```python
from build123d import *

# Parameters (mm, degrees)
SKETCH_1_W              = 50
SKETCH_1_H              = 100
SKETCH_1_R              = 6.25
EXTRUDE_1_DEPTH         = 16
HOLE_WIZARD_M16_1_D     = 14
HOLE_WIZARD_M16_1_DEPTH = 38
HOLE_WIZARD_M16_1_TIP   = 4.206024333
SKETCH_5_R              = 9.25
CUT_EXTRUDE_1_DEPTH     = 12


with BuildPart() as part:
    # 草图1 → 凸台-拉伸1 (new body)
    with BuildSketch(Plane(origin=(0, 0, 0), x_dir=(1, 0, 0), z_dir=(0, 1, 0))):
        with Locations((25, 50)):
            Rectangle(SKETCH_1_W, SKETCH_1_H)
        with Locations(Location((25, 75, 0), (0, 0, 270))):
            Circle(SKETCH_1_R, mode=Mode.SUBTRACT)
        with Locations(Location((25, 25, 0), (0, 0, 270))):
            Circle(SKETCH_1_R, mode=Mode.SUBTRACT)
    extrude(amount=EXTRUDE_1_DEPTH)

    # M16 螺纹孔1
    with Locations(Plane(origin=(25, 16, -50), x_dir=(0, 0, 1), z_dir=(0, 1, 0))):
        with Locations((0, 0)):
            Hole(HOLE_WIZARD_M16_1_D / 2, depth=HOLE_WIZARD_M16_1_DEPTH)
            with Locations((0, 0, -(HOLE_WIZARD_M16_1_DEPTH + HOLE_WIZARD_M16_1_TIP / 2))):  # 118° drill point
                Cone(0, HOLE_WIZARD_M16_1_D / 2, HOLE_WIZARD_M16_1_TIP, mode=Mode.SUBTRACT)

    # 草图5 → 切除-拉伸1 (cut)
    with BuildSketch(Plane.XZ):
        with Locations(Location((25, -25, 0), (0, 0, 270))):
            Circle(SKETCH_5_R)
        with Locations(Location((25, -75, 0), (0, 0, 270))):
            Circle(SKETCH_5_R)
    extrude(amount=-CUT_EXTRUDE_1_DEPTH, mode=Mode.SUBTRACT)


solid = part.part
```
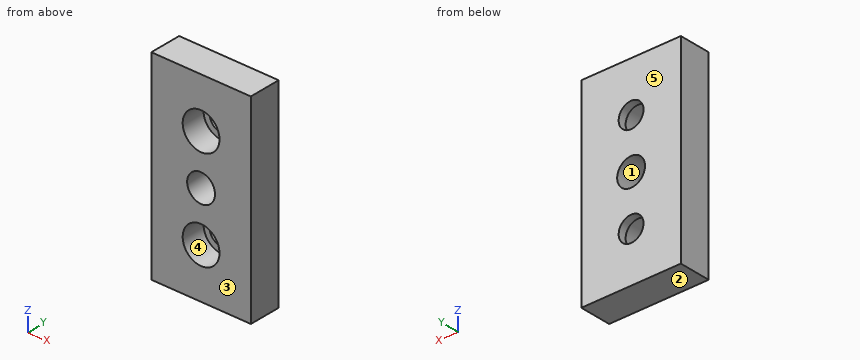
Model file for the job. Use its own axes, mm. Face numbers are marked on the shaded views. A direction names the side the tool comes from. Coordinates: 2 decimals unless noted, no trailing zeros. Order: outer loops, then holes, each group sorted by start corner. A loop starts at its lowest first (then second) coordinate and runs counter-clockwise, first axis right, second up. Notation, with made-up numbers: (-4.5, -33.75) -> (5.5, -33.75) arc R16 cw to (5.5, -11.75) -> close; hole circle Ø1 at (36.25, 16). An arc over 180 degrees is marked (long way). Answer as a JSON object with one key per item and string values. Group by question number.
1) Cut at C-C, the plane y = 10.5. Write the cut outline in (x, z), then the cut area to 3 significant figures.
2) Cut at B-B, the plane x = 25. Write the cut outline in (y, z), then the cut area to 3 significant figures.
3) Which spindle directions (+Z, -Z, +X, -X, +Y, -Y) get a long thin tool onto all of the face, cutting with end or side? Do the marked faces 4 and 5. Say none if no direction does.
4) Flat gauge pins, fed straight in: pin 1 (12.5 mm diameter, centred on x = 25, z = -50, fed in from -Y); pin 2 (9 mm diameter, centred on x = 26.5, z = -26, fed in from -Y). Where does each tip first touch, or does it go through?
5) Drill centre lines: L1, parallel to X at y = 9.5, z = -50; L2, parallel to X at y = 14.9, z = -25; L3, parallel to Y at x = 33, z = -71. Where is each one in solid material? Low to high.
6) Pull direction Z, two halves, no side cores. Call the marked faces 1, 2 and 3: +Z half, -Z half, draft (parallel to the pull), parting line (faces both ways), or undercut.
7) Cut at D-D, the plane z = -50. Write the cut outline in (x, y).
8) Cut at A-A, the plane z = -25. Write the cut outline in (x, y).
Check values:
{
 "1": {"outline": "(0, -100) -> (50, -100) -> (50, 0) -> (0, 0) -> close; hole circle Ø18.5 at (25, -75); hole circle Ø18.5 at (25, -25); hole circle Ø14 at (25, -50)", "area": "4,310 mm²"},
 "2": {"outline": "(0, -100) -> (16, -100) -> (16, -81.25) -> (12, -81.25) -> (12, -84.25) -> (0, -84.25) -> close; (0, -65.75) -> (12, -65.75) -> (12, -68.75) -> (16, -68.75) -> (16, -57) -> (0, -57) -> close; (0, -43) -> (16, -43) -> (16, -31.25) -> (12, -31.25) -> (12, -34.25) -> (0, -34.25) -> close; (0, -15.75) -> (12, -15.75) -> (12, -18.75) -> (16, -18.75) -> (16, 0) -> (0, 0) -> close", "area": "832 mm²"},
 "3": {"face 4": "-Y", "face 5": "+Z, -Z, +X, -X, +Y"},
 "4": {"pin 1": "passes through", "pin 2": "stops at y = 12"},
 "5": {"L1": "x = 0 to 18, 32 to 50", "L2": "x = 0 to 18.75, 31.25 to 50", "L3": "y = 12 to 16"},
 "6": {"face 1": "undercut", "face 2": "-Z half", "face 3": "draft"},
 "7": {"outline": "(0, 0) -> (18, 0) -> (18, 16) -> (0, 16) -> close; (32, 0) -> (50, 0) -> (50, 16) -> (32, 16) -> close"},
 "8": {"outline": "(0, 0) -> (15.75, 0) -> (15.75, 12) -> (18.75, 12) -> (18.75, 16) -> (0, 16) -> close; (31.25, 12) -> (34.25, 12) -> (34.25, 0) -> (50, 0) -> (50, 16) -> (31.25, 16) -> close"}
}
